```python
from build123d import *

# Parameters (mm, degrees)
BOSS_EXTRUDE1_DEPTH = 12.5
BOSS_EXTRUDE2_DEPTH = 6
SKETCH4_R           = 2.5
BOSS_EXTRUDE3_DEPTH = 3
SKETCH5_R           = 1.25
CUT_EXTRUDE1_DEPTH  = 2.6


with BuildPart() as part:
    # Sketch2 → Boss-Extrude1 (new body)
    with BuildSketch(Plane.YZ):
        Polygon((0, 0), (0, 18), (-4.75, 18), (-4.75, 20.6), (0, 20.6), (0, 22.5), (22.7, 22.5), (22.7, 20.6), (27.45, 20.6), (27.45, 18), (22.7, 18), (22.7, 0), align=None)
    extrude(amount=BOSS_EXTRUDE1_DEPTH)

    # Sketch3 → Boss-Extrude2 (add)
    with BuildSketch(Plane.XY.offset(22.5)):
        with BuildLine():
            ThreePointArc((2.778708958, 11.252631579), (3.938700525, 9.071712585), (6.25, 8.2))
            Line((6.25, 8.2), (6.25, 10.2))
            ThreePointArc((6.25, 10.2), (4.436309375, 10.468944381), (2.778708958, 11.252631579))
        make_face()
        with BuildLine():
            Line((6.25, 10.2), (6.25, 8.2))
            ThreePointArc((6.25, 8.2), (8.561299475, 9.071712585), (9.721291042, 11.252631579))
            ThreePointArc((9.721291042, 11.252631579), (8.063690625, 10.468944381), (6.25, 10.2))
        make_face()
        with BuildLine():
            ThreePointArc((2.778708958, 11.252631579), (4.436309375, 10.468944381), (6.25, 10.2))
            Line((6.25, 10.2), (6.25, 15.2))
            ThreePointArc((6.25, 15.2), (3.621712585, 14.011299475), (2.778708958, 11.252631579))
        make_face()
        with BuildLine():
            Line((6.25, 15.2), (6.25, 10.2))
            ThreePointArc((6.25, 10.2), (8.063690625, 10.468944381), (9.721291042, 11.252631579))
            ThreePointArc((9.721291042, 11.252631579), (9.742815386, 11.475855678), (9.75, 11.7))
            ThreePointArc((9.75, 11.7), (8.724873734, 14.174873734), (6.25, 15.2))
        make_face()
        with BuildLine():
            ThreePointArc((6.25, 22.7), (0.268944381, 18.263690625), (2.778708958, 11.252631579))
            ThreePointArc((2.778708958, 11.252631579), (3.621712585, 14.011299475), (6.25, 15.2))
            Line((6.25, 15.2), (6.25, 22.7))
        make_face()
        with BuildLine():
            ThreePointArc((9.75, 11.7), (9.742815386, 11.475855678), (9.721291042, 11.252631579))
            ThreePointArc((9.721291042, 11.252631579), (11.761717927, 13.503227953), (12.5, 16.45))
            ThreePointArc((12.5, 16.45), (10.669417382, 20.869417382), (6.25, 22.7))
            Line((6.25, 22.7), (6.25, 15.2))
            ThreePointArc((6.25, 15.2), (8.724873734, 14.174873734), (9.75, 11.7))
        make_face()
    extrude(amount=BOSS_EXTRUDE2_DEPTH)

    # Sketch4 → Boss-Extrude3 (add)
    with BuildSketch(Plane.XY.offset(28.5)):
        with Locations((6.25, 16.45)):
            Circle(SKETCH4_R)
    extrude(amount=BOSS_EXTRUDE3_DEPTH)

    # Sketch5 → Cut-Extrude1 (cut)
    with BuildSketch(Plane.XY.offset(20.6)):
        with BuildLine():
            Line((7, 27.45), (5.5, 27.45))
            Line((5.5, 27.45), (5.5, 26.2))
            ThreePointArc((5.5, 26.2), (6.25, 26.45), (7, 26.2))
            Line((7, 26.2), (7, 27.45))
        make_face()
        with Locations((6.25, 25.2)):
            Circle(SKETCH5_R)
        with BuildLine():
            ThreePointArc((7, -3.5), (6.25, -3.75), (5.5, -3.5))
            Line((5.5, -3.5), (5.5, -4.75))
            Line((5.5, -4.75), (7, -4.75))
            Line((7, -4.75), (7, -3.5))
        make_face()
        with Locations((6.25, -2.5)):
            Circle(SKETCH5_R)
    extrude(amount=-CUT_EXTRUDE1_DEPTH, mode=Mode.SUBTRACT)


solid = part.part
```
CAD build for the part. Positions are in the model's coordinates, mm. A direction names the side the tool comes from. Round coordinates to 2 decimals unless told otherwise and drop trailing zeros. Loops run counter-clockwise (first coordinate to the right, second up) from the corner with the lowest first, then second, coordinate; pieces in that order, holes last. Notation, with made-up numbers: M 70,44.25 L 114,44.25 A14 ccw 114,68.25 Z; hole C -19,70.5 d8. An arc over 180 degrees is marked long. Return JSON: item names as keys, results as strings. Group by question number.
(1) Tool access for faces 5 (the flat face through (5.5, -4, 19)), 6 (the flat face through (4.8, -2.4, 20.6)), 7 (the flat face through (8, 14, 28.5)), 8 (the flat face through (7, 27, 19)): list every direction of +Z, -Z, +X, -X, +Y, -Y with a clear straight run to the whole face (end or side of a thin tool).
(2) Mould opens along Y. For faces 1 (the cylindrical face through (6.21, 23.95, 19.32)), 2 (the flat face through (6, 22.7, 22)), 3 (the flat face through (3, -4.75, 19)), 4 (the flat face through (6, 12, 0)) say: +Y half, -Y half, draft (parallel to the pull), parting line (faces both ways), or undercut.
(3) Wall check: probe 1 along X at (y, z) = (-2.5, 19.2); probe 2 along Y at (x, z) = (6.25, 18.9); probe 3 along Z at (x, y) = (6.75, 12). Give the ranges that are in metal, low to high. Write a range as [from, to].
(4) Saw through at B-B, the plane z = 20. List the corners of the cut face in (x, y), and give its area (3 significant figures).
(5) Drop flat-ended pins along their axis: P1, Ø4, axis at x = 6.25, y = 25.2, coming from the -Z side; P2, Ø1, axis at x = 3.5, y = 3.5, coming from the +Z side; P3, Ø3, axis at x = 1.5, y = 19.5, coming from the +Z side. Give the stop position or say it passes through.
(6) Saw through at A-A, the plane y = -2.5. List the corners of the cut face in (x, z), and give its area (3 significant figures).
(7) Saw through at C-C, the plane y = 18. List the corners of the cut face in (x, z).
(8) Saw through at D-D, the plane x = 4.25. List the corners of the cut face in (y, z), and give its area (3 significant figures).
Answer list:
{
 "1": {"face 5": "+Z, -Z, -Y", "face 6": "+Z, +X, -X, -Y", "face 7": "+Z", "face 8": "+Z, -Z, +Y"},
 "2": {"face 1": "undercut", "face 2": "+Y half", "face 3": "-Y half", "face 4": "draft"},
 "3": {"probe 1": "[0, 5], [7.5, 12.5]", "probe 2": "[-1.25, 23.95]", "probe 3": "[0, 28.5]"},
 "4": {"outline": "M 0,-4.75 L 5.5,-4.75 L 5.5,-3.5 A1.25 cw long 7,-3.5 L 7,-4.75 L 12.5,-4.75 L 12.5,27.45 L 7,27.45 L 7,26.2 A1.25 cw long 5.5,26.2 L 5.5,27.45 L 0,27.45 Z", "area": "389 mm2"},
 "5": {"P1": "z = 18", "P2": "z = 22.5", "P3": "z = 28.5"},
 "6": {"outline": "M 0,18 L 5,18 L 5,20.6 L 0,20.6 Z; M 7.5,18 L 12.5,18 L 12.5,20.6 L 7.5,20.6 Z", "area": "26.0 mm2"},
 "7": {"outline": "M 0,0 L 12.5,0 L 12.5,22.5 L 12.3,22.5 L 12.3,28.5 L 8.21,28.5 L 8.21,31.5 L 4.29,31.5 L 4.29,28.5 L 0.2,28.5 L 0.2,22.5 L 0,22.5 Z"},
 "8": {"outline": "M -4.75,18 L 0,18 L 0,0 L 22.7,0 L 22.7,18 L 27.45,18 L 27.45,20.6 L 22.7,20.6 L 22.7,22.5 L 22.37,22.5 L 22.37,28.5 L 17.95,28.5 L 17.95,31.5 L 14.95,31.5 L 14.95,28.5 L 8.83,28.5 L 8.83,22.5 L 0,22.5 L 0,20.6 L -4.75,20.6 Z", "area": "626 mm2"}
}
